Model file for the job. Use its own axes, mm. A direction names the side the tool comes from. Give positions to 0.01 mm unless a question says otherwise; leave off trailing zeros. Loops run counter-clockwise (first coordinate to the right, second up) from the corner with the lowest first, then second, coordinate; pieces in that order, holes last. Notation, with made-up numbers: M 65.25,-26 L 77.25,-26 A25 cw 77.25,-4 Z; hole C -15.75,22.5 d1. An arc over 180 degrees is marked long. Answer in a Markdown table with one row per item.
```python
from build123d import *

# Parameters (mm, degrees)
F1_DEPTH = 49
F2_W     = 4.3
F2_H     = 15
F3_DEPTH = 25
F4_W     = 4.85
F4_H     = 2.7
F5_DEPTH = 1.8
F6_R     = 2
F7_SIZE2 = 1.4281480067
F7_SIZE  = 1
F9_DEPTH = 38


with BuildPart() as f1:
    # F0 (on Top) → F1 (new body)
    with BuildSketch(Plane.XY):
        Polygon((-3.075, -9.3), (-3.075, 0), (0, 0), (3.075, 0), (3.075, -9.3), (7, -9.3), (7, 2.7), (0, 2.7), (-7, 2.7), (-7, -9.3), align=None)
    extrude(amount=F1_DEPTH)

    # F2 (on face) → F3 (cut)
    with BuildSketch(Plane(origin=(0, 2.7, 0), x_dir=(-1, 0, 0), z_dir=(0, 1, 0))):
        with Locations((0, 7.5)):
            Rectangle(F2_W, F2_H)
    extrude(amount=-F3_DEPTH, mode=Mode.SUBTRACT)

    # F4 (on face) → F5 (join)
    with BuildSketch(Plane(origin=(0, 0, 0), x_dir=(1, 0, 0), z_dir=(0, 0, -1))):
        Polygon((2.15, -2.7), (7, -2.7), (7, 0), (3.075, 0), (2.15, 0), align=None)
        with Locations((-4.575, -1.35)):
            Rectangle(F4_W, F4_H)
    extrude(amount=F5_DEPTH)

    # F6
    f6_edges = [f1.edges().sort_by_distance(p)[0] for p in [
        (2.15, 1.35, 15),
        (-2.15, 1.35, 15),
    ]]
    fillet(f6_edges, radius=F6_R)

    # F7
    f7_edges = [f1.edges().sort_by_distance(p)[0] for p in [
        (4.575, 2.7, -1.8),
        (-4.575, 2.7, -1.8),
    ]]
    f7_side = f1.faces().sort_by_distance((0, 2.7, 25.492605))[0]
    chamfer(f7_edges, length=F7_SIZE, length2=F7_SIZE2, reference=f7_side)

    # F8 (on face) → F9 (cut)
    with BuildSketch(Plane.XY.offset(49)):
        Polygon((7, -3.3), (7, 1.4), (5.5, 1.4), (5.5, -0.7019237886), align=None)
        Polygon((-5.5, 1.4), (-7, 1.4), (-7, -3.3), (-5.5, -0.7019237886), align=None)
    extrude(amount=-F9_DEPTH, mode=Mode.SUBTRACT)


solid = f1.part
```
Q1. Probe probe 1 along X at (y, z) = (-3.5, 29.5) (3 decimals); probe 2 along X at (y, z) = (-0.5, 41.5) (3 decimals); probe 3 along Y at (x, z) = (-2.5, 22.5). List the from-to ranges inside material, lowest first.
Reported:
| item | result |
|---|---|
| probe 1 | -7 to -3.075, 3.075 to 7 |
| probe 2 | -5.5 to -3.075, 3.075 to 5.5 |
| probe 3 | 0 to 2.7 |
Q2. Mould opens along X. For faces 6 (the face through (7, -5, 18)), 7 (the face through (6, 1.4, 30)), 8 (the face through (3.075, -5, 24)) say: released by +X, released by -X, zero draft, split by the parting line, or undercut.
Reported:
| item | result |
|---|---|
| face 6 | released by +X |
| face 7 | zero draft |
| face 8 | undercut |
Q3. Saw through at C-C (x = -4.25). Give the cut face in (y, z), and give its area (3 significant figures).
Reported:
| item | result |
|---|---|
| outline | M -9.3,0 L 0,0 L 0,-1.8 L 1.27,-1.8 L 2.7,-0.8 L 2.7,49 L -9.3,49 Z |
| area | 592 mm² |
Q4. Saw through at A-A (y = -7.25). Give the cut face in (x, z) (3 decimals).
Reported:
| item | result |
|---|---|
| outline | M -7,0 L -3.075,0 L -3.075,49 L -7,49 Z; M 3.075,0 L 7,0 L 7,49 L 3.075,49 Z |
Q5. Saw through at D-D (z = 14.5). Give the cut face in (x, y) (3 decimals), and give its area (3 significant figures).
Reported:
| item | result |
|---|---|
| outline | M -7,-9.3 L -3.075,-9.3 L -3.075,0 L -1.473,0 L -1.473,2.7 L -7,2.7 L -7,1.4 L -5.5,1.4 L -5.5,-0.702 L -7,-3.3 Z; M 1.473,0 L 3.075,0 L 3.075,-9.3 L 7,-9.3 L 7,-3.3 L 5.5,-0.702 L 5.5,1.4 L 7,1.4 L 7,2.7 L 1.473,2.7 Z |
| area | 92.6 mm² |
Q6. 3-axis set-ups, long thin cutter, end or side, ignore diameter. For faces 1 (the face through (-2.15, 1, 5)), 2 (the face through (-5, -9.3, 24)), 3 (the face through (-5.5, 0, 30)), 4 (the face through (-5, -5, 0)), 5 (the face through (6.24, -1.98, 30.27)): which of +Z, -Z, +X, -X, +Y, -Y reach the whole face in a straight line?
Reported:
| item | result |
|---|---|
| face 1 | -Z, +Y, -Y |
| face 2 | +Z, -Z, +X, -X, -Y |
| face 3 | +Z, -X |
| face 4 | -Z, +X, -X, -Y |
| face 5 | +Z, +X |
Q7. Drop flat-ended pins along their axis: pin 1 (1.7 mm diameter, centred on y = 0.5, z = 33, fed in from -X); pin 2 (2 mm diameter, centred on x = -2.5, y = -5, fed in from +Z); pin 3 (2 mm diameter, centred on x = -2.5, y = -8, fed in from -Z). Give the stop position or say it passes through.
Reported:
| item | result |
|---|---|
| pin 1 | x = -5.5 |
| pin 2 | z = 49 |
| pin 3 | z = 0 |
Q8. Saw through at B-B (z = 39). Give the cut face in (x, y) (3 decimals), and give its area (3 significant figures).
Reported:
| item | result |
|---|---|
| outline | M -7,-9.3 L -3.075,-9.3 L -3.075,0 L 3.075,0 L 3.075,-9.3 L 7,-9.3 L 7,-3.3 L 5.5,-0.702 L 5.5,1.4 L 7,1.4 L 7,2.7 L -7,2.7 L -7,1.4 L -5.5,1.4 L -5.5,-0.702 L -7,-3.3 Z |
| area | 101 mm² |
